Could you check a few things on this model? Use its own coordinates, in mm. Coordinates: 2 decimals unless noted, no trailing zeros. Loops run counter-clockwise (first coordinate to the right, second up) from the corner with the lowest first, then second, coordinate; pieces in that order, holes last. Notation, with made-up numbers: (-19.5, 75.25) - (-9.5, 75.25) arc R24 cw to (-9.5, 91.25) - close; hole circle Ø11 at (-34, 29.5). An arc over 180 degrees is marked (long way). Use CSV: the item, a comma, the result in double quotes.
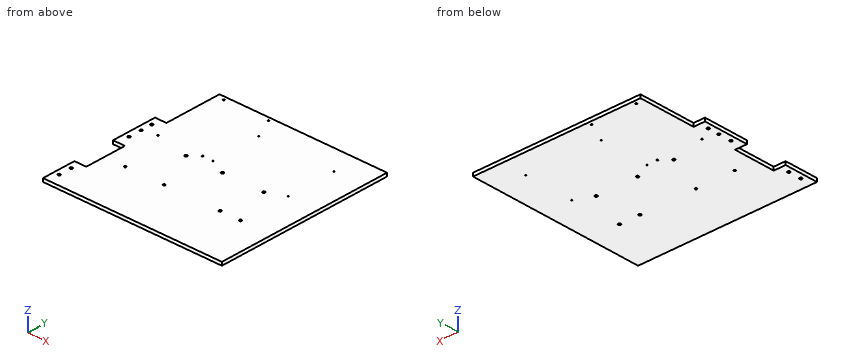
from build123d import *

# Parameters (mm, degrees)
MODEL_R             = 2.5
MODEL_R_2           = 2
MODEL_R_3           = 1.5
MODEL_R_4           = 1.05
BOSS_EXTRUDE1_DEPTH = 6.35


with BuildPart() as part:
    # Model → Boss-Extrude1 (new body)
    with BuildSketch(Plane.XY):
        Polygon((731.320358487, 258.065863271), (386.320358487, 258.065863271), (386.320358487, 323.065863271), (409.320358487, 323.065863271), (409.320358487, 403.065863271), (386.320358487, 403.065863271), (386.320358487, 490.065863271), (408.320358487, 490.065863271), (408.320358487, 600.065863271), (731.320358487, 600.065863271), align=None)
        with Locations((396.320358487, 472.687351768)):
            Circle(MODEL_R, mode=Mode.SUBTRACT)
        with Locations((396.320358487, 450.687351768)):
            Circle(MODEL_R, mode=Mode.SUBTRACT)
        with Locations((396.320358487, 425.687351768)):
            Circle(MODEL_R, mode=Mode.SUBTRACT)
        with Locations((396.320358487, 305.687351768)):
            Circle(MODEL_R, mode=Mode.SUBTRACT)
        with Locations((396.320358487, 280.687351768)):
            Circle(MODEL_R, mode=Mode.SUBTRACT)
        with Locations((491.320358487, 441.687351768)):
            Circle(MODEL_R, mode=Mode.SUBTRACT)
        with Locations((561.320358487, 441.687351768)):
            Circle(MODEL_R, mode=Mode.SUBTRACT)
        with Locations((641.320358487, 441.687351768)):
            Circle(MODEL_R, mode=Mode.SUBTRACT)
        with Locations((449.26902181, 360.687351768)):
            Circle(MODEL_R_2, mode=Mode.SUBTRACT)
        with Locations((524.320358487, 360.687351768)):
            Circle(MODEL_R_2, mode=Mode.SUBTRACT)
        with Locations((423.320358487, 592.687351768)):
            Circle(MODEL_R_3, mode=Mode.SUBTRACT)
        with Locations((509.320358487, 592.687351768)):
            Circle(MODEL_R_3, mode=Mode.SUBTRACT)
        with Locations((509.320358487, 456.687351768)):
            Circle(MODEL_R_3, mode=Mode.SUBTRACT)
        with Locations((423.320358487, 456.687351768)):
            Circle(MODEL_R_3, mode=Mode.SUBTRACT)
        with Locations((529.320358487, 551.687351768)):
            Circle(MODEL_R_4, mode=Mode.SUBTRACT)
        with Locations((674.320358487, 551.687351768)):
            Circle(MODEL_R_4, mode=Mode.SUBTRACT)
        with Locations((529.320358487, 456.687351768)):
            Circle(MODEL_R_4, mode=Mode.SUBTRACT)
        with Locations((674.320358487, 456.687351768)):
            Circle(MODEL_R_4, mode=Mode.SUBTRACT)
        with Locations((631.970358487, 361.072616848)):
            Circle(MODEL_R, mode=Mode.SUBTRACT)
        with Locations((671.320358487, 361.072616848)):
            Circle(MODEL_R, mode=Mode.SUBTRACT)
    extrude(amount=-BOSS_EXTRUDE1_DEPTH)


solid = part.part
(1) Will these pins go through, and if not, where does the flat tip stop? pin 1 (3.5 mm diameter, centred on x = 529.32, y = 551.69, fed in from +Z); pin 2 (1.9 mm diameter, centred on x = 400, z = -3.5, fed in from +Y); pin 3 (3 mm diameter, centred on y = 545, z = -1.5, fed in from -X).
Computed:
pin 1,"stops at z = 0"
pin 2,"stops at y = 490.07"
pin 3,"stops at x = 408.32"
(2) Suppose I cut it at A-A (z = -3.25). State how many separate pieces and enclosed holes the cut face has, plus the area to 3 significant figures.
Computed:
separate pieces,"1"
enclosed holes,"20"
area,"113,000 mm²"
(3) Suppose I cut it at B-B (y = 351.5). Write out the boundary of the cut face in (x, z).
Computed:
outline,"(409.32, -6.35) - (731.32, -6.35) - (731.32, 0) - (409.32, 0) - close"
(4) Suppose I cut it at C-C (y = 508.5). Write out the boundary of the cut face in (x, z).
Computed:
outline,"(408.32, -6.35) - (731.32, -6.35) - (731.32, 0) - (408.32, 0) - close"
(5) Please list where these lines run through material, in increasing order: line 1 (X direction, y = 473, z = -3.5); line 2 (Y direction, x = 406.5, z = -1); line 3 (Y direction, x = 524.5, z = -4).
Computed:
line 1,"x = 386.32 to 393.84, 398.8 to 731.32"
line 2,"y = 258.07 to 323.07, 403.07 to 490.07"
line 3,"y = 258.07 to 358.7, 362.68 to 600.07"
